Autodesk Inventor part; units mm, degrees
ref_plane "YZ Plane" through (0, 0, 0) normal (1, 0, 0) x (0, 1, 0)
ref_plane "XZ Plane" through (0, 0, 0) normal (0, 1, 0) x (-1, 0, 0)
ref_plane "XY Plane" through (0, 0, 0) normal (0, 0, 1) x (1, 0, 0)
sketch "Sketch1" plane through (0, 0, 0) normal (0, 1, 0) x (-1, 0, 0)
  line L0 (0, -2) -> (0, -12.5)
  line L1 (0, -12.5) -> (-3, -12.5)
  line L2 (-2, 0) -> (-12.5, 0)
  line L3 (-12.5, 0) -> (-12.5, -3)
  line L4 (-12.5, -3) -> (-3.1, -3)
  line L5 (-3, -3.1) -> (-3, -12.5)
  line L6 (0, 0) -> (-12.1249, -12.1249) construction
  arc A0 (-3, -3.1) -> (-3.1, -3) centre (-3.1, -3.1) ccw
  arc A1 (0, -2) -> (-2, 0) centre (-2, -2) ccw
  line L7 (-15.0828, 0) -> (2.9971, 0)
  point P0 (-3, -3)
  dimension "d4" = 3
  dimension "d8" = 0.1
  dimension "d9" = 2
  dimension "d16" = 90
  dimension "d17" = 12.5
extrude "Extrusion1" add sketch "Sketch1" along normal blind 15
sketch "Sketch2" plane through (0, 15, 0) normal (0, 1, 0) x (1, 0, 0)
  line L0 (0, 12.5) -> (0, 2)
  line L1 (2, 0) -> (12.5, 0)
  line L2 (12.5, 0) -> (12.5, 3)
  line L3 (12.5, 3) -> (3.1, 3)
  line L4 (3, 3.1) -> (3, 12.5)
  line L5 (3, 12.5) -> (0, 12.5)
  line L6 (12.5, 3) -> (3, 12.5)
  arc A0 (0, 2) -> (2, 0) centre (2, 2) ccw
  arc A1 (3, 3.1) -> (3.1, 3) centre (3.1, 3.1) ccw
  point P0 (0, 0)
extrude "Extrusion2" add sketch "Sketch2" along normal blind 3
sketch "Sketch3" plane through (12.5, 0, -3) normal (0, 0, -1) x (-1, 0, 0)
  line L0 (0, 0) -> (9.4, 0)
  line L1 (0, 0) -> (0, 15)
  circle A0 centre (4.7, 7.5) radius 1.5
  line L2 (9.4, 0) -> (9.4, 15)
  line L3 (0, 15) -> (9.4, 15)
  point P0 (12.5, 0)
  point P1 (4.7, 0)
  point P2 (0, 7.5)
  dimension "d5" = 3
extrude "Extrusion3" cut sketch "Sketch3" against normal through all contours A0
sketch "Sketch5" plane through (3, 0, -12.5) normal (1, 0, 0) x (0, 0, -1)
  circle A0 centre (-4.7, 7.5) radius 1.5
  line L0 (-9.4, 0) -> (0, 0)
  line L1 (0, 0) -> (0, 15)
  line L2 (-9.4, 15) -> (0, 15)
  line L3 (-9.4, 0) -> (-9.4, 15)
  point P0 (-12.5, 0)
  point P1 (0, 7.5)
  dimension "d12" = 3
  dimension "d18" = 4.7
extrude "Extrusion4" cut sketch "Sketch5" against normal through all contours A0
fillet "Fillet1" radius 1.5 2 edges at (1.5, 0, -12.5) (12.5, 0, -1.5)
properties part number "EE_adapter_forOld"
Work out the finished part from the listing and answer in its coordinate system (mm). A direction names the side the tool comes from. Give positions to 0.01 mm unless a question says otherwise; leave off trailing zeros. Loops run counter-clockwise (first coordinate to the right, second up) from the corner with the lowest first, then second, coordinate; pieces in that order, holes last. Notation, with made-up numbers: (63.5, 28.5) -> (87.5, 28.5) arc R30 cw to (87.5, 63.5) -> close; hole circle Ø5 at (85, 46). An arc over 180 degrees is marked (long way). Use a Markdown table: item, result. Add a question column.
1) The part is cut by section D-D, the plane z = -4. Determine the outline of the cut face in (x, y).
2) Which of the six approach directions +Z, -Z, +X, -X, +Y, -Y give full straight-line access (tool end or side, diameter ignored) to faces 4 (the flat face through (3, 5.7, -7.7)), 5 (the cylindrical face through (12.07, 0.45, -1.52))?
3) Consider line 1 along Y through (x, z) = (7.8, -2.35); line 2 along X through (y, z) = (10.25, -10); line 3 along Z through (x, y) = (10.5, 7.5). Determine where each line is inside the solid, lowest interval first.
4) The part is cut by section A-A, the plane y = 7.5. Determine the outline of the cut face in (x, z).
5) Each of these flat-tipped pins is pushed along its axis until it touches: P1, Ø7.5, axis at x = 6.5, z = -5.5, coming from the -Y side; P2, Ø4.5, axis at y = 7, z = -7.5, coming from the +X side; P3, Ø6, axis at x = 11, y = 15, coming from the -Z side; P4, Ø2, axis at x = 5.5, z = -7.5, coming from the -Y side. Where does it stop, or does it pass through?
6) The part is cut by section C-C, the plane z = -7.8. Determine the outline of the cut face in (x, y), plus the area to 3 significant figures.
7) For a pull along Y with two mould halves and no side action, classify faces 1 (the flat face through (4, 0, -2)), 2 (the flat face through (5, 18, -5)), 3 (the cylindrical face through (9, 6.6, -1.5)) as +Y half, -Y half, draft (parallel to the pull), parting line (faces both ways), or undercut.
8) The part is cut by section B-B, the plane x = 7.8. Determine the outline of the cut face in (y, z).
Reported:
| question | item | result |
|---|---|---|
| 1 | outline | (0, 0) -> (3, 0) -> (3, 15) -> (11.5, 15) -> (11.5, 18) -> (0, 18) -> close |
| 2 | face 4 | -Z, +X, -Y |
| 2 | face 5 | +Z, -Z, +X, -Y |
| 3 | line 1 | y = 0 to 6, 9 to 18 |
| 3 | line 2 | x = 0 to 3 |
| 3 | line 3 | z = -3 to 0 |
| 4 | outline | (0, -12.5) -> (3, -12.5) -> (3, -9.3) -> (0, -9.3) -> close; (0, -6.3) -> (3, -6.3) -> (3, -3.1) arc R0.1 cw to (3.1, -3) -> (6.3, -3) -> (6.3, 0) -> (2, 0) arc R2 ccw to (0, -2) -> close; (9.3, -3) -> (12.5, -3) -> (12.5, 0) -> (9.3, 0) -> close |
| 5 | P1 | stops at y = 0 |
| 5 | P2 | stops at x = 3 |
| 5 | P3 | stops at z = -7.5 |
| 5 | P4 | stops at y = 15 |
| 6 | outline | (0, 0) -> (3, 0) -> (3, 6) -> (0, 6) -> close; (0, 9) -> (3, 9) -> (3, 15) -> (7.7, 15) -> (7.7, 18) -> (0, 18) -> close |
| 6 | area | 59.1 mm^2 |
| 7 | face 1 | -Y half |
| 7 | face 2 | +Y half |
| 7 | face 3 | undercut |
| 8 | outline | (0, -3) -> (6, -3) -> (6, 0) -> (0, 0) -> close; (9, -3) -> (15, -3) -> (15, -7.7) -> (18, -7.7) -> (18, 0) -> (9, 0) -> close |
